For this review, take the finished solid that the model builds, in its own axes (mm). Face numbers are marked on the shaded views. A direction names the side the tool comes from. Coordinates: 2 decimals unless noted, no trailing zeros. Loops run counter-clockwise (first coordinate to the right, second up) from the corner with the lowest first, then second, coordinate; pieces in that order, holes last. Notation, with made-up numbers: (24.25, 65) - (49.25, 65) arc R31 ccw to (49.25, 95) - close; hole circle Ø6 at (69, -36.75). An arc over 180 degrees is marked (long way). Answer as a JSON object with one key per item and string values. Group by question number.
Item 1: To check wall thickness, follow line 1 (Y direction, x = -683.5, z = 5); line 2 (X direction, y = 90, z = 2.5); line 3 (X direction, y = 91.5, z = 0.5). State the ranges of each line that lie inside material, in increasing order.
Item 2: Mouldability with a two-part tool opening along X and no side actions: class the marked faces 4, 5 and 6 as released by +X, released by -X, zero draft, split by the parting line, or undercut.
Item 3: Tool access review of the marked faces 1, 2 and 3: name each direction out of +Z, -Z, +X, -X, +Y, -Y from which nothing blocks a thin tool from reaching the whole face with its end or side.
Item 4: We need section C-C (x = -664). Give the boundary of the cut face in (y, z), then the cut area to 3 significant figures.
Item 5: Clearance check with flat-ended pins moving along their axes: pin 1 (2 mm diameter, centred on x = -679, z = 2.5, fed in from -Y); pin 2 (1.4 mm diameter, centred on x = -685.5, z = 3.5, fed in from +Y); pin 3 (2.5 mm diameter, centred on x = -686.43, z = 3.18, fed in from -Y). State where each tip first meets the part, or that it passes through.
Item 6: We need section A-A (x = -685.5). Give the boundary of the cut face in (y, z), then the cut area to 3 significant figures.
Item 7: We need section B-B (x = -655.5). Give the boundary of the cut face in (y, z), then the cut area to 3 significant figures.
from build123d import *

# Parameters (mm, degrees)
BOSS_EXTRUDE1_DEPTH                            = 6.35
FILLET1_R                                      = 0.508
CBORE_FOR_4_SOCKET_HEAD_CAP_SCREW1_D           = 2.9464
CBORE_FOR_4_SOCKET_HEAD_CAP_SCREW1_CBORE_D     = 4.826
CBORE_FOR_4_SOCKET_HEAD_CAP_SCREW1_CBORE_DEPTH = 2.8448
TAP_DRILL_FOR_4_40_TAP1_D                      = 2.2606
TAP_DRILL_FOR_4_40_TAP1_DEPTH                  = 7.357911993
TAP_DRILL_FOR_4_40_TAP1_TIP                    = 0.679152758
TAP_DRILL_FOR_4_40_TAP2_D                      = 2.2606
TAP_DRILL_FOR_4_40_TAP2_DEPTH                  = 8.235563733
TAP_DRILL_FOR_4_40_TAP2_TIP                    = 0.679152758


with BuildPart() as part:
    # Model → Boss-Extrude1 (new body)
    with BuildSketch(Plane.XY):
        with BuildLine():
            Line((-662.928291328, 76.124043703), (-690.700357042, 76.124043703))
            Line((-690.700357042, 76.124043703), (-690.700357042, 82.474043703))
            Line((-690.700357042, 82.474043703), (-682.661678057, 82.474043703))
            ThreePointArc((-682.661678057, 82.474043703), (-680.416614026, 82.474043703), (-680.416614026, 84.719107734))
            Line((-680.416614026, 84.719107734), (-680.416614026, 99.844571929))
            Line((-680.416614026, 99.844571929), (-637.431275221, 66.6046705))
            ThreePointArc((-637.431275221, 66.6046705), (-636.837083068, 64.625922801), (-638.517578145, 63.42407295))
            Line((-638.517578145, 63.42407295), (-660.683227297, 63.42407295))
            Line((-660.683227297, 63.42407295), (-660.683227297, 73.878979673))
            ThreePointArc((-660.683227297, 73.878979673), (-660.683227297, 76.124043703), (-662.928291328, 76.124043703))
        make_face()
    extrude(amount=BOSS_EXTRUDE1_DEPTH)

    # Fillet1
    fillet1_edges = [part.edges().sort_by_distance(p)[0] for p in [
        (-690.700357042, 76.124043703, 3.175),
        (-690.700357042, 82.474043703, 3.175),
        (-680.416614026, 99.844571929, 3.175),
        (-660.683227297, 63.42407295, 3.175),
    ]]
    fillet(fillet1_edges, radius=FILLET1_R)

    # CBORE for #4 Socket Head Cap Screw1 (through all)
    with Locations(Plane(origin=(0, 82.474043703, 0), x_dir=(1, 0, 0), z_dir=(0, 1, 0))):
        with Locations((-686.427017549, -3.175)):
            CounterBoreHole(CBORE_FOR_4_SOCKET_HEAD_CAP_SCREW1_D / 2, CBORE_FOR_4_SOCKET_HEAD_CAP_SCREW1_CBORE_D / 2, CBORE_FOR_4_SOCKET_HEAD_CAP_SCREW1_CBORE_DEPTH)

    # Tap Drill for #4-40 Tap1
    with Locations(Plane(origin=(-206.299258714, -266.783087499, 0), x_dir=(0.7910716317479708, -0.6117235269659022, 0), z_dir=(0.6117235269659022, 0.7910716317479708, 0))):
        with Locations((-555.88255935, -3.175)):
            Hole(TAP_DRILL_FOR_4_40_TAP1_D / 2, depth=TAP_DRILL_FOR_4_40_TAP1_DEPTH)
            with Locations((0, 0, -(TAP_DRILL_FOR_4_40_TAP1_DEPTH + TAP_DRILL_FOR_4_40_TAP1_TIP / 2))):  # 118° drill point
                Cone(0, TAP_DRILL_FOR_4_40_TAP1_D / 2, TAP_DRILL_FOR_4_40_TAP1_TIP, mode=Mode.SUBTRACT)

    # Tap Drill for #4-40 Tap2
    with Locations(Plane(origin=(-206.299258714, -266.783087499, 0), x_dir=(0.7910716317479708, -0.6117235269659022, 0), z_dir=(0.6117235269659022, 0.7910716317479708, 0))):
        with Locations((-587.63255935, -3.175)):
            Hole(TAP_DRILL_FOR_4_40_TAP2_D / 2, depth=TAP_DRILL_FOR_4_40_TAP2_DEPTH)
            with Locations((0, 0, -(TAP_DRILL_FOR_4_40_TAP2_DEPTH + TAP_DRILL_FOR_4_40_TAP2_TIP / 2))):  # 118° drill point
                Cone(0, TAP_DRILL_FOR_4_40_TAP2_D / 2, TAP_DRILL_FOR_4_40_TAP2_TIP, mode=Mode.SUBTRACT)


solid = part.part
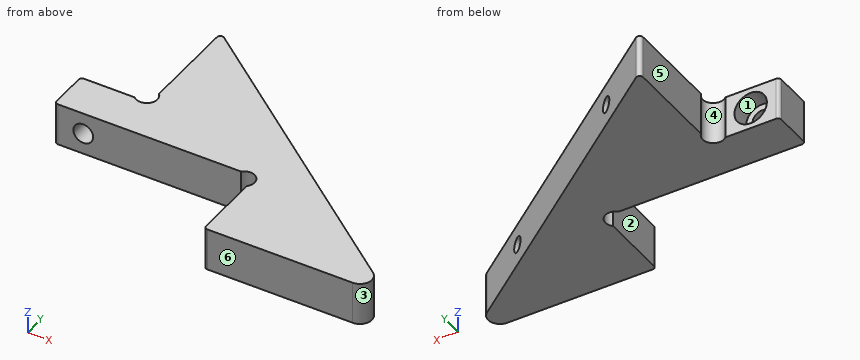
Check sheet entries:
{
 "1": {"line 1": "y = 76.12 to 82.47", "line 2": "x = -680.42 to -674.38, -672.09 to -667.69", "line 3": "x = -680.42 to -669.63"},
 "2": {"face 4": "undercut", "face 5": "released by -X", "face 6": "zero draft"},
 "3": {"face 1": "+Y", "face 2": "+Z, -Z, -X, -Y", "face 3": "+Z, -Z, +X"},
 "4": {"outline": "(76.12, 0) - (87.15, 0) - (87.15, 6.35) - (76.12, 6.35) - close", "area": "70.0 mm2"},
 "5": {"pin 1": "stops at y = 76.12", "pin 2": "stops at y = 79.63", "pin 3": "passes through"},
 "6": {"outline": "(76.12, 0) - (82.47, 0) - (82.47, 0.95) - (79.63, 0.95) - (79.63, 2.03) - (76.12, 2.03) - close; (76.12, 4.32) - (79.63, 4.32) - (79.63, 5.4) - (82.47, 5.4) - (82.47, 6.35) - (76.12, 6.35) - close", "area": "19.6 mm2"},
 "7": {"outline": "(63.42, 0) - (80.58, 0) - (80.58, 6.35) - (63.42, 6.35) - close", "area": "109 mm2"}
}
